from build123d import *

# Parameters (mm, degrees)
F0_W          = 23
F0_H          = 6.4641016151
F1_DEPTH      = 51
F2_T          = -1.5
F3_DEPTH      = 18
F4_DEPTH      = 18
F5_T          = -1
F6_W          = 9.5
F6_H          = 4
F7_DEPTH      = 3
F8_DEPTH      = 1
F8_DEPTH_BACK = 2
F10_DEPTH     = 25
F6_W_2        = 2
F6_H_2        = 5
F11_DEPTH     = 1


with BuildPart() as f1:
    # F0 (on Right) → F1 (new body)
    with BuildSketch(Plane.YZ):
        with Locations((-7.2324005883, 2.3867851467)):
            Rectangle(F0_W, F0_H)
        Polygon((-5.4682982052, 28.5929351986), (-18.7324005883, 5.6188359543), (4.2675994117, 5.6188359543), (4.2675994117, 20.9285051598), align=None)
        Polygon((4.2675994117, 20.9285051598), (4.2675994117, 5.6188359543), (4.2675994117, -0.8452656608), (24.2675994117, -0.8452656608), (24.2675994117, 5.1838243087), align=None)
    extrude(amount=-F1_DEPTH)

    # F2
    f2_openings = [f1.faces().sort_by_distance(p)[0] for p in [
        (-25.5, -12.100349, 17.105886),
    ]]
    offset(amount=F2_T, openings=f2_openings)

    # F0 (on Right) → F3 (cut)
    with BuildSketch(Plane.YZ):
        Polygon((4.2675994117, 20.9285051598), (4.2675994117, 5.6188359543), (4.2675994117, -0.8452656608), (24.2675994117, -0.8452656608), (24.2675994117, 5.1838243087), align=None)
    extrude(amount=-F3_DEPTH, mode=Mode.SUBTRACT)

    # F6 (on face) → F7 (cut)
    with BuildSketch(Plane.XZ.offset(18.7324005883)):
        Polygon((-5, -0.1132148533), (-5, 4.8867851467), (-15, 4.8867851467), (-15, 4.3867851467), (-5.5, 4.3867851467), (-5.5, 0.3867851467), (-15, 0.3867851467), (-15, -0.1132148533), align=None)
        with Locations((-10.25, 2.3867851467)):
            Rectangle(F6_W, F6_H)
    extrude(amount=-F7_DEPTH, mode=Mode.SUBTRACT)

    # F6 (on face) → F8 (join, two sides)
    with BuildSketch(Plane.XZ.offset(18.7324005883)) as f8_sk:
        with Locations((-10.25, 2.3867851467)):
            Rectangle(F6_W, F6_H)
    extrude(amount=-F8_DEPTH)
    extrude(f8_sk.sketch, amount=F8_DEPTH_BACK)

    # F9 (on face) → F10 (cut)
    with BuildSketch(Plane.XY.offset(4.3867851467)):
        Polygon((-15, -18.7324005883), (-15, -20.7324005883), (-7.75, -20.7324005883), (-10.25, -18.7324005883), align=None)
    extrude(amount=-F10_DEPTH, mode=Mode.SUBTRACT)



with BuildPart() as f4:
    # F0 (on Right) → F4 (new body)
    with BuildSketch(Plane.YZ):
        Polygon((4.2675994117, 20.9285051598), (4.2675994117, 5.6188359543), (4.2675994117, -0.8452656608), (24.2675994117, -0.8452656608), (24.2675994117, 5.1838243087), align=None)
    extrude(amount=-F4_DEPTH)

    # F5
    f5_openings = [f4.faces().sort_by_distance(p)[0] for p in [
        (0, 12.379942, 6.848464),
    ]]
    offset(amount=F5_T, openings=f5_openings)


with BuildPart() as f1_1:
    add(f1.part)

    add(f4.part)  # F11 merges F4
    # F6 (on face) → F11 (join)
    with BuildSketch(Plane.XZ.offset(18.7324005883)):
        with Locations((-1, 2.3867851467)):
            Rectangle(F6_W_2, F6_H_2)
    extrude(amount=F11_DEPTH)


solid = f1_1.part
Verification items for the finished model (mm, model axes). A direction names the side the tool comes from. Give positions to 0.01 mm unless a question says otherwise; leave off trailing zeros. Write each loop counter-clockwise with the first axis right and the second up, starting at its lowest first coordinate (ties: lowest second). Pieces come first, ordered by that corner, then holes.
(1) Material ranges on line 1 (X direction, y = 22, z = 2); line 2 (Y direction, x = -39.5, z = 2.5); line 3 (Y direction, x = -11, z = 3.75), recorded low to high.
(2) Cross-section at A-A (x = -6.5). Enter the section's corners in (y, z), plus the area to 3 significant figures.
(3) Gauge pin test, flat ends, axial feed: pin 1 (1.5 mm diameter, centred on x = -34.5, z = 7, fed in from +Y); pin 2 (5 mm diameter, centred on x = -33, z = 3.5, fed in from -Y); pin 3 (1 mm diameter, centred on x = -0.5, z = 3, fed in from -Y); pin 4 (3.5 mm diameter, centred on y = -17.5, z = 2.5, fed in from +X). Record the tip position at first contact, or that the pin passes through.
(4) Access from +Z, -Z, +X, -X, +Y, -Y to the whole of each face (thin tool, end or side, straight path). Record for faces 1 (the face through (-18, 11, 8)), 2 (the face through (-10, -18, 4.887)), 3 (the face through (-25, -17.232, 4)), 4 (the face through (-8.381, 14.394, 11.684)).
(5) Cross-section at B-B (y = 10). Enter the section's corners in (x, z).
(6) Cross-section at D-D (x = -41.5). Enter the section's corners in (y, z).
(7) Cross-section at C-C (z = 1.75). Enter the section's corners in (x, y), plus the area to 3 significant figures.
(8) Mould release check, pull along Y, two halves, no side actions. Record for faces 5 (the face through (-10, -17.732, 2)), 6 (the face through (-51, 2, 11)), 7 (the face through (-1, -19.732, 2)): +Y half, -Y half, draft (parallel to the pull), parting line (faces both ways), or undercut.
Worked out:
1. line 1: x = -51 to -49.5, -18 to -17
1. line 2: y = -18.73 to -17.23, 22.77 to 24.27
1. line 3: y = -18.73 to -17.73, 4.27 to 5.27, 23.27 to 24.27
2. outline: (-20.73, 0.39) - (-17.73, 0.39) - (-17.73, 4.39) - (-20.73, 4.39) - close; (-18.73, -0.85) - (24.27, -0.85) - (24.27, 5.18) - (-5.47, 28.59) - (-6.23, 27.28) - (4.27, 19.02) - (4.27, 0.65) - (-15.73, 0.65) - (-15.73, -0.11) - (-18.73, -0.11) - close; (-18.73, 4.89) - (-17.23, 4.89) - (-17.23, 8.22) - (-18.73, 5.62) - close; hole (5.27, 0.15) - (23.27, 0.15) - (23.27, 4.7) - (5.27, 18.87) - close
2. area: 135 mm2
3. pin 1: stops at y = 22.91
3. pin 2: stops at y = -18.73
3. pin 3: stops at y = -19.73
3. pin 4: stops at x = 0
4. face 1: none
4. face 2: -Y
4. face 3: +Z
4. face 4: +X
5. outline: (-51, -0.85) - (0, -0.85) - (0, 0.15) - (-17, 0.15) - (-17, 15.14) - (0, 15.14) - (0, 16.42) - (-51, 16.42) - close; hole (-49.5, 0.65) - (-18, 0.65) - (-18, 14.51) - (-49.5, 14.51) - close
6. outline: (-18.73, -0.85) - (24.27, -0.85) - (24.27, 5.18) - (-5.47, 28.59) - (-6.23, 27.28) - (22.77, 4.46) - (22.77, 0.65) - (-17.23, 0.65) - (-17.23, 8.22) - (-18.73, 5.62) - close
7. outline: (-51, -18.73) - (-10.25, -18.73) - (-7.75, -20.73) - (-5.5, -20.73) - (-5.5, -17.73) - (-15, -17.73) - (-15, -17.23) - (-49.5, -17.23) - (-49.5, 22.77) - (-18, 22.77) - (-18, 4.27) - (-1.5, 4.27) - (-1.5, -17.23) - (-5, -17.23) - (-5, -18.73) - (-2, -18.73) - (-2, -19.73) - (0, -19.73) - (0, 5.27) - (-17, 5.27) - (-17, 23.27) - (0, 23.27) - (0, 24.27) - (-51, 24.27) - close
7. area: 276 mm2
8. face 5: undercut
8. face 6: draft
8. face 7: -Y half
